For this review, take the finished solid that the model builds, in its own axes (mm). Round coordinates to 2 decimals unless told otherwise and drop trailing zeros. Order: outer loops, then holes, each group sorted by start corner. A loop starts at its lowest first (then second) coordinate and runs counter-clockwise, first axis right, second up.
from build123d import *

# Parameters (mm, degrees)
BOSS_EXTRUDE1_DEPTH = 5.2832
CHAMFER1_SIZE       = 3.81
CHAMFER2_SIZE       = 3.81


with BuildPart() as part:
    # Sketch1 → Boss-Extrude1 (new body)
    with BuildSketch(Plane(origin=(0, 0, 0), x_dir=(1, 0, 0), z_dir=(0, 1, 0))):
        Polygon((0, 0), (203.2, 0), (157.48, 67.056), (76.2, 67.056), align=None)
    extrude(amount=BOSS_EXTRUDE1_DEPTH)

    # Chamfer1
    # the kernel refuses this chamfer: 3.81 mm, written as the material it takes off along each edge
    with BuildSketch(Plane(origin=(83.555575257, 5.2832, -73.528906226), x_dir=(-0.018164543083463394, -0.9996219169112968, -0.020641526231208396), z_dir=(-0.7507135169227552, 0, 0.6606278948920248))) as chamfer1_piece_1:
        Polygon((CHAMFER1_SIZE * 0.999621916911, CHAMFER1_SIZE * 0.0274958766106), (-CHAMFER1_SIZE * 0.0274958766106, CHAMFER1_SIZE * 0.999621916911), (0, 0), align=None)
    extrude(amount=121.099658478, mode=Mode.SUBTRACT)
    with BuildSketch(Plane(origin=(83.555575257, 0, -73.528906226), x_dir=(-0.018164543083463394, 0.9996219169112968, -0.020641526231208396), z_dir=(-0.7507135169227552, 0, 0.6606278948920248))) as chamfer1_piece_2:
        Polygon((CHAMFER1_SIZE * 0.999621916911, -CHAMFER1_SIZE * 0.0274958766106), (-CHAMFER1_SIZE * 0.0274958766106, -CHAMFER1_SIZE * 0.999621916911), (0, 0), align=None)
    extrude(amount=121.099658478, mode=Mode.SUBTRACT)

    # Chamfer2
    # the kernel refuses this chamfer: 3.81 mm, written as the material it takes off along each edge
    with BuildSketch(Plane(origin=(208.719637405, 0, 8.095468194), x_dir=(-0.8259149602218081, -0.027495876610586452, 0.5631238365148687), z_dir=(-0.5633368246415095, 0, -0.8262273428075478)), Plane(origin=(208.719637405, 5.2832, 8.095468194), x_dir=(0.022717845070130322, -0.9996219169112966, -0.015489439820543389), z_dir=(-0.5633368246415095, 0, -0.8262273428075478))) as chamfer2_piece_1:
        Polygon((CHAMFER2_SIZE * 0.999621916911, CHAMFER2_SIZE * 0.0274958766106), (-CHAMFER2_SIZE * 0.0274958766106, CHAMFER2_SIZE * 0.999621916911), (0, 0), align=None)
    extrude(amount=100.75548469, mode=Mode.SUBTRACT)


solid = part.part
(1) Add section D-D on z = -52. Give the boundary of the cut face in (x, y).
(2) Clearance check with flat-ended pins moving along their axes: P1, Ø2, axis at y = 4.5, z = -18.5, coming from the -X side; P2, Ø1, axis at y = 1.5, z = -44, coming from the -X side. State where each tip first meets the part, or that it passes through.
(3) Wall thickness on L1, parallel to X at y = 4.9, z = -26.5; L2, parallel to X at y = 1.55, z = -22; L3, parallel to Z at x = 75.5, y = 4.25: over which ranges is each line inside the solid? List them lowest first.
(4) Add section B-B on z = -13. Give the boundary of the cut face in (x, y).
(5) Add section C-C on y = 3.75. Give the boundary of the cut face in (x, z), plus the area to 3 significant figures.
(6) Add section A-A on x = 48. Give the boundary of the cut face in (y, z).
Here are the results:
1. outline: (60.86, 2.64) - (64.86, 0) - (163.13, 0) - (166.33, 2.64) - (163.13, 5.28) - (64.86, 5.28) - close
2. P1: stops at x = 23.71
2. P2: stops at x = 52.55
3. L1: x = 35.3 to 180.98
3. L2: x = 28.42 to 185.46
3. L3: z = -62.74 to 0
4. outline: (16.54, 2.64) - (20.54, 0) - (189.73, 0) - (192.92, 2.64) - (189.73, 5.28) - (20.54, 5.28) - close
5. outline: (3.45, 0) - (79.65, -67.06) - (154.72, -67.06) - (200.44, 0) - close
5. area: 9,120 mm2
6. outline: (0, -37.16) - (2.64, -40.68) - (5.28, -37.16) - (5.28, 0) - (0, 0) - close
